```python
from build123d import *

# Parameters (mm, degrees)
SKETCH_2_W      = 2
SKETCH_2_H      = 20
SKETCH_2_W_2    = 50
SKETCH_2_H_2    = 2
SKETCH_2_W_3    = 135
SKETCH_2_H_3    = 60
EXTRUDE_1_DEPTH = 2


with BuildPart() as part:
    # 草图2 → 凸台-拉伸1 (new body)
    with BuildSketch(Plane(origin=(0, 0, 0), x_dir=(1, 0, 0), z_dir=(0, 1, 0))):
        with Locations((-1, 0)):
            Rectangle(SKETCH_2_W, SKETCH_2_H)
        with Locations((65, 31)):
            Rectangle(SKETCH_2_W_2, SKETCH_2_H_2)
        with Locations((136, 0)):
            Rectangle(SKETCH_2_W, SKETCH_2_H)
        with Locations((65, -31)):
            Rectangle(SKETCH_2_W_2, SKETCH_2_H_2)
        with Locations((67.5, 0)):
            Rectangle(SKETCH_2_W_3, SKETCH_2_H_3)
    extrude(amount=EXTRUDE_1_DEPTH)


solid = part.part
```
For this review, take the finished solid that the model builds, in its own axes (mm). Coordinates: 2 decimals unless noted, no trailing zeros. Write each loop counter-clockwise with the first axis right and the second up, starting at its lowest first coordinate (ties: lowest second). Pieces come first, ordered by that corner, then holes. Notation, with made-up numbers: (26.25, 60) - (44.25, 60) arc R13 ccw to (44.25, 85) - close; hole circle Ø9 at (-33.5, -4). An arc over 180 degrees is marked (long way). Answer in a Markdown table with one row per item. Add a question column.
Q1. For probe 1 along X at (y, z) = (0.7, -23); probe 2 along Z at (x, y) = (30.5, 1.2), list the stretches that pass through material, from the lowest coordinate up.
Q2. For P1, Ø0.6, axis at y = 1.5, z = 15, coming from the -X side; P2, Ø1, axis at x = 116.5, y = 1.5, coming from the -Z side; P3, Ø0.6, axis at x = -1, y = 1, coming from the -Z side, all flat-tipped, find the tip position at first contact; note any pin that passes through.
Q3. We need section A-A, the plane y = 0.4. State the section outline as (x, z) points, and give its area (3 significant figures).
Q4. We need section C-C, the plane z = -23. State the section outline as (x, y) points, and give its area (3 significant figures).
Q5. We need section B-B, the plane x = 114. State the section outline as (y, z) points, and give its area (3 significant figures).
Answer list:
| question | item | result |
|---|---|---|
| 1 | probe 1 | x = 0 to 135 |
| 1 | probe 2 | z = -30 to 30 |
| 2 | P1 | stops at x = 0 |
| 2 | P2 | stops at z = -30 |
| 2 | P3 | stops at z = -10 |
| 3 | outline | (-2, -10) - (0, -10) - (0, -30) - (40, -30) - (40, -32) - (90, -32) - (90, -30) - (135, -30) - (135, -10) - (137, -10) - (137, 10) - (135, 10) - (135, 30) - (90, 30) - (90, 32) - (40, 32) - (40, 30) - (0, 30) - (0, 10) - (-2, 10) - close |
| 3 | area | 8,380 mm2 |
| 4 | outline | (0, 0) - (135, 0) - (135, 2) - (0, 2) - close |
| 4 | area | 270 mm2 |
| 5 | outline | (0, -30) - (2, -30) - (2, 30) - (0, 30) - close |
| 5 | area | 120 mm2 |
